from build123d import *

# Parameters (mm, degrees)
F0_R     = 889
F1_DEPTH = 914.4
F0_R_2   = 209.55
F2_DEPTH = 25.4


with BuildPart() as f1:
    # F0 (on Front) → F1 (new body)
    with BuildSketch(Plane.XZ):
        Circle(F0_R)
        with BuildLine():
            ThreePointArc((-586.1689197433, 599.1537678485), (325.0018857416, 772.6273450147), (838.2, 0))
            ThreePointArc((838.2, 0), (-325.0018857416, -772.6273450147), (-586.1689197433, 599.1537678485))
        make_face(mode=Mode.SUBTRACT)
    extrude(amount=F1_DEPTH)

    # F0 (on Front) → F2 (join)
    with BuildSketch(Plane.XZ):
        Circle(F0_R)
        with BuildLine():
            ThreePointArc((-586.1689197433, 599.1537678485), (325.0018857416, 772.6273450147), (838.2, 0))
            ThreePointArc((838.2, 0), (-325.0018857416, -772.6273450147), (-586.1689197433, 599.1537678485))
        make_face(mode=Mode.SUBTRACT)
        with BuildLine():
            ThreePointArc((-586.1689197433, 599.1537678485), (-325.0018857416, -772.6273450147), (838.2, 0))
            ThreePointArc((838.2, 0), (325.0018857416, 772.6273450147), (-586.1689197433, 599.1537678485))
        make_face()
        with Locations((-112.8989619291, -403.6070296654)):
            Circle(F0_R_2, mode=Mode.SUBTRACT)
        with BuildLine():
            ThreePointArc((-146.5422299358, 149.7884419621), (-442.8729018337, 153.0346539884), (-439.6266898075, 449.3653258863))
            ThreePointArc((-439.6266898075, 449.3653258863), (-211.8339884362, 492.7337201779), (-83.5344598716, 299.5768839242))
            ThreePointArc((-83.5344598716, 299.5768839242), (-99.927623618, 218.3264124888), (-146.5422299358, 149.7884419621))
        make_face(mode=Mode.SUBTRACT)
        with Locations((405.9834218008, 104.0301457412)):
            Circle(F0_R_2, mode=Mode.SUBTRACT)
    extrude(amount=-F2_DEPTH)


solid = f1.part
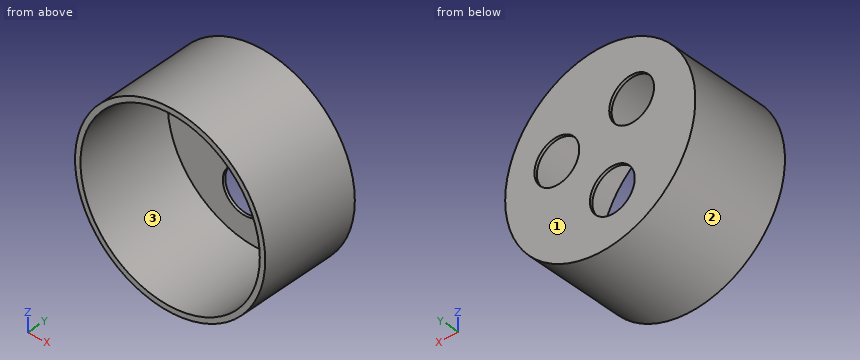
Verification items for the finished model (mm, model axes). Face numbers are marked on the shaded views. Give positions to 0.01 mm unless a question says otherwise; leave off trailing zeros. Loops run counter-clockwise (first coordinate to the right, second up) from the corner with the lowest first, then second, coordinate; pieces in that order, holes last. Notation, with made-up numbers: (81, 25.5) - (117, 25.5) arc R21 cw to (117, 49.5) - close; hole circle Ø2 at (53, 78.25). An arc over 180 degrees is marked (long way). Write item = value, one per line. Start each with the question number.
Q1. Cross-section at A-A, the plane z = -438. Enter the section's corners in (x, y), and give its area (3 significant figures).
Q2. Cross-section at C-C, the plane z = 240. Enter the section's corners in (x, y), and give its area (3 significant figures).
Q3. Cross-section at D-D, the plane x = 654. Enter the section's corners in (y, z).
Q4. Thickness scan on line 1 (Z direction, x = 0, y = -564); line 2 (Y direction, x = -95.5, z = -619); line 3 (X direction, y = -571, z = -24.5). Record the ranges inside material, lowest first.
Q5. Mould release check, pull along Z, two halves, no side actions. Record for the marked faces 1, 2 and 3: released by +Z, released by -Z, zero draft, split by the parting line, or undercut.
Q6. Depth check by flat-ended pin: P1, Ø1, axis at y = -409.5, z = 575.5, coming from the +X side; P2, Ø1.5, axis at y = -289, z = -595.5, coming from the +X side; P3, Ø8, axis at x = -160, y = -293.5, coming from the -Z side. Enter the tip coordinate at first touch or a pass-through.
Q7. Cross-section at B-B, the plane x = 0. Enter the section's corners in (y, z), and give its area (3 significant figures).
Answer key:
q1.outline = (-773.61, -914.4) - (-714.66, -914.4) - (-714.66, 0) - (-319.61, 0) - (-319.61, 25.4) - (-773.61, 25.4) - close; (93.81, 0) - (714.66, 0) - (714.66, -914.4) - (773.61, -914.4) - (773.61, 25.4) - (93.81, 25.4) - close
q1.area = 137,000 mm^2
q2.outline = (-855.99, -914.4) - (-803.11, -914.4) - (-803.11, 0) - (-493.99, 0) - (-493.99, 25.4) - (-855.99, 25.4) - close; (-92.18, 0) - (246.54, 0) - (246.54, 25.4) - (-92.18, 25.4) - close; (565.43, 0) - (803.11, 0) - (803.11, -914.4) - (855.99, -914.4) - (855.99, 25.4) - (565.43, 25.4) - close
q2.area = 122,000 mm^2
q3.outline = (-914.4, -602.17) - (25.4, -602.17) - (25.4, 602.17) - (-914.4, 602.17) - (-914.4, 524.27) - (0, 524.27) - (0, -524.27) - (-914.4, -524.27) - close
q4.line_1 = -889 to -838.2, 838.2 to 889
q4.line_2 = 0 to 25.4
q4.line_3 = -888.66 to -837.84, 837.84 to 888.66
q5.face_1 = zero draft
q5.face_2 = split by the parting line
q5.face_3 = undercut
q6.P1 = 678.01
q6.P2 = 660.75
q6.P3 = -875.21
q7.outline = (-914.4, -889) - (25.4, -889) - (25.4, -580.14) - (0, -580.14) - (0, -838.2) - (-914.4, -838.2) - close; (-914.4, 838.2) - (0, 838.2) - (0, -227.07) - (25.4, -227.07) - (25.4, 889) - (-914.4, 889) - close
q7.area = 129,000 mm^2
